Part print with two shaded views. Sizes in mm from the minimum x, y, z corner. A direction names the side the tool comes from. Give positions to 0.01 mm unless a question says otherwise; leave off trailing zeros. Order: outer loops, then holes, each group sorted by start corner. A loop starts at its lowest first (then second) coordinate and runs counter-clockwise, first axis right, second up. Notation, with made-up numbers: M 23.5,19 L 62.5,19 A22 ccw 62.5,42 Z; hole C -23.5,23.25 d5. An arc over 180 degrees is marked long. Return JSON: item names as keys, results as strings.
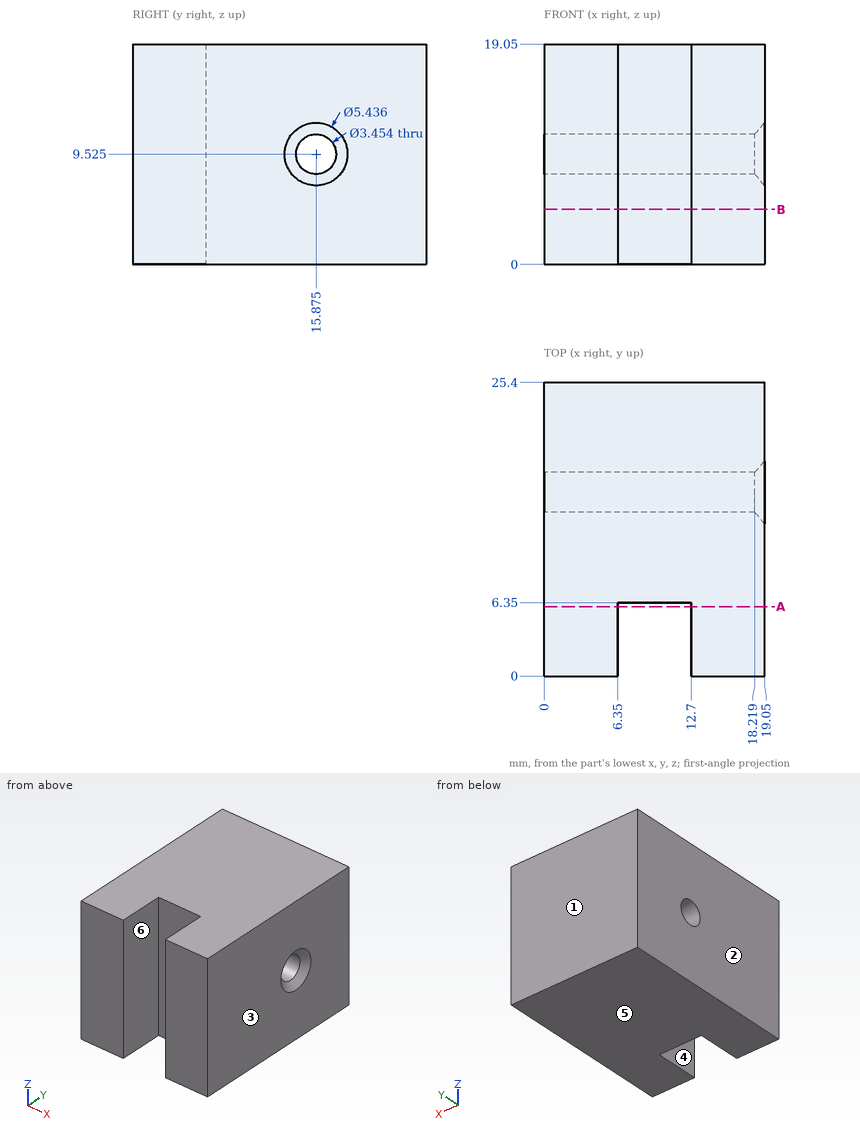
Q1. Two-plate mould, pull along X, no slides. Class the marked faces 1, 2, 3 and 4: +X half, -X half, draft (parallel to the pull), parting line (faces both ways), or undercut.
Established:
{"face 1": "draft", "face 2": "-X half", "face 3": "+X half", "face 4": "undercut"}
Q2. Band-saw the part on A-A (y = 6). Give the cut face in (x, z).
Established:
{"outline": "M 0,0 L 6.35,0 L 6.35,19.05 L 0,19.05 Z; M 12.7,0 L 19.05,0 L 19.05,19.05 L 12.7,19.05 Z"}
Q3. Pin check, flat tip, straight feed: pin 1 (1.9 mm diameter, centred on x = 10.5, z = 13, fed in from -Y). Stop position of the tip, or through.
Established:
{"pin 1": "stops at y = 6.35"}
Q4. Band-saw the part on B-B (z = 4.75). Give the cut face in (x, y).
Established:
{"outline": "M 0,0 L 6.35,0 L 6.35,6.35 L 12.7,6.35 L 12.7,0 L 19.05,0 L 19.05,25.4 L 0,25.4 Z"}
Q5. 3-axis set-ups, long thin cutter, end or side, ignore diameter. For the marked faces 5 and 6: which of +Z, -Z, +X, -X, +Y, -Y reach the whole face in a straight line?
Established:
{"face 5": "-Z, +X, -X, +Y, -Y", "face 6": "+Z, -Z, -Y"}
Q6. Probe line 1 along Z through (x, y) = (17, 16); line 2 along X through (y, z) = (6, 16.75); line 3 along Y through (x, z) = (12.5, 2.75). List the from-to ranges inside material, lowest first.
Established:
{"line 1": "z = 0 to 7.8, 11.25 to 19.05", "line 2": "x = 0 to 6.35, 12.7 to 19.05", "line 3": "y = 6.35 to 25.4"}
